from build123d import *

# Parameters (mm, degrees)
BOSS_EXTRUDE1_DEPTH = 5.08
CUT_EXTRUDE1_DEPTH  = 155.095804696
LPATTERN1_COUNT     = 28
LPATTERN1_PITCH     = 9.974326
SKETCH4_W           = 279.4
SKETCH4_H           = 25.4
BOSS_EXTRUDE2_DEPTH = 7.62


with BuildPart() as part:
    # Sketch1 → Boss-Extrude1 (new body)
    with BuildSketch(Plane(origin=(0, 0, 0), x_dir=(1, 0, 0), z_dir=(0, 1, 0))):
        Polygon((-149.225, -38.1), (-149.225, 28.194), (130.175, 28.194), (130.175, 12.954), (-130.175, 12.954), (-130.175, 0), (130.175, 0), (130.175, -38.1), align=None)
    extrude(amount=BOSS_EXTRUDE1_DEPTH)

    # Sketch2 → Cut-Extrude1 (cut, through all)
    with BuildSketch(Plane(origin=(0, 5.08, 0), x_dir=(1, 0, 0), z_dir=(0, 1, 0))):
        with BuildLine():
            ThreePointArc((-146.56997683, 19.717013973), (-147.330155915, 24.13319761), (-149.225, 28.194))
            ThreePointArc((-149.225, 28.194), (-144.836574415, 28.369434802), (-140.448148829, 28.194))
            ThreePointArc((-140.448148829, 28.194), (-142.342992915, 24.13319761), (-143.103171999, 19.717013973))
            ThreePointArc((-143.103171999, 19.717013973), (-144.836574415, 19.749434802), (-146.56997683, 19.717013973))
        make_face()
    cut_extrude1 = extrude(amount=-CUT_EXTRUDE1_DEPTH, mode=Mode.SUBTRACT)

    # LPattern1: Cut-Extrude1 ×28
    with Locations(*[(i * LPATTERN1_PITCH, 0, 0) for i in range(1, LPATTERN1_COUNT)]):
        add(cut_extrude1, mode=Mode.SUBTRACT)

    # Sketch4 → Boss-Extrude2 (add)
    with BuildSketch(Plane.XZ):
        with Locations((-9.525, 25.4)):
            Rectangle(SKETCH4_W, SKETCH4_H)
    extrude(amount=BOSS_EXTRUDE2_DEPTH)


solid = part.part
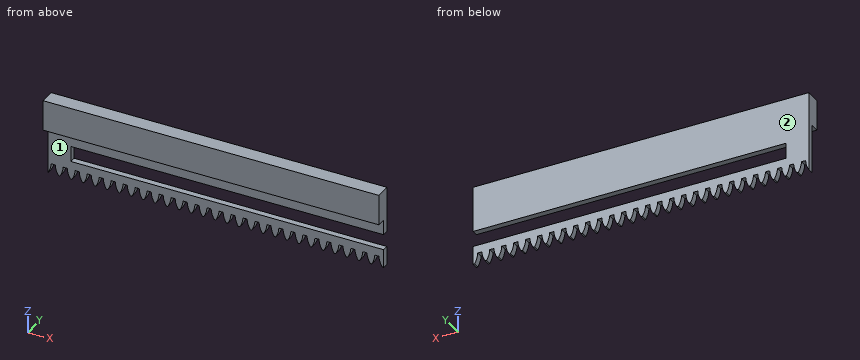
Model file for the job. Use its own axes, mm. Face numbers are marked on the shaded views. A direction names the side the tool comes from. Give positions to 0.01 mm unless a question says otherwise; leave off trailing zeros. Order: outer loops, then holes, each group sorted by start corner. A loop starts at its lowest first (then second) coordinate and runs counter-clockwise, first axis right, second up. Notation, with made-up numbers: (85.25, 8) -> (93.25, 8) arc R29 cw to (93.25, 30) -> close; hole circle Ø7 at (89.25, 35). An arc over 180 degrees is marked (long way). Use CSV: the item, a comma, the result in double quotes.
1. Drop flat-ended pins along their axis: pin 1 (4 mm diameter, centred on x = 6.5, y = 3.5, fed in from -Z); pin 2 (5 mm diameter, centred on x = -20, z = 4.5, fed in from -Y); pin 3 (4 mm diameter, centred on y = 3.5, z = -5.5, fed in from +X) (3 decimals); pin 4 (6 mm diameter, centred on y = -4, z = -6, fed in from -X). Give the stop position or say it passes through.
Outcome:
pin 1,"z = -27.06"
pin 2,"y = 0"
pin 3,"x = -130.175"
pin 4,"through"
2. Band-saw the part on B-B, the plane z = -6. Give the cut face in (x, y) (3 decimals), then the cut area to 3 significant figures.
Outcome:
outline,"(-149.225, 0) -> (-130.175, 0) -> (-130.175, 5.08) -> (-149.225, 5.08) -> close"
area,"96.8 mm²"
3. Band-saw the part on A-A, the plane z = 9. Give the cut face in (x, y) (3 decimals).
Outcome:
outline,"(-149.225, 0) -> (130.175, 0) -> (130.175, 5.08) -> (-149.225, 5.08) -> close"
4. Drill centre lines: line 1 along Z through (x, y) = (79, 1.25); line 2 along Y through (x, z) = (-32, 8); line 3 along Z through (x, y) = (-76.5, -4). Where is each one in solid material? Low to high. Write a range as from..to.
Outcome:
line 1,"-28.19..-12.95, 0..38.1"
line 2,"0..5.08"
line 3,"12.7..38.1"
5. 3-axis set-ups, long thin cutter, end or side, ignore diameter. For the marked faces 1 and 2: which of +Z, -Z, +X, -X, +Y, -Y reach the whole face in a straight line?
Outcome:
face 1,"-Z, +X, -X, -Y"
face 2,"+Z, -Z, +X, -X, +Y"
